```python
from build123d import *

# Parameters (mm, degrees)
SKETCH002_R        = 9.5
SKETCH002_R_2      = 4.05
PAD_DEPTH          = 1
PAD001_DEPTH       = 7
PAD002_DEPTH       = 3
POLARPATTERN_COUNT = 3


with BuildPart() as part:
    # Sketch002 → Pad (new body)
    with BuildSketch(Plane.XY):
        Circle(SKETCH002_R)
        Circle(SKETCH002_R_2, mode=Mode.SUBTRACT)
    extrude(amount=PAD_DEPTH)

    # Sketch003 (on Face4 of Pad) → Pad001 (join)
    with BuildSketch(Plane.XY.offset(1)):
        with BuildLine():
            ThreePointArc((4.0493831654, 0.0706822461), (3.5759377511, 1.9013598293), (2.3229845672, 3.3175657794))
            Line((5.4489761453, 7.7819444208), (2.3229845672, 3.3175657794))
            ThreePointArc((9.498553104, 0.1657978612), (8.3880021321, 4.4599798465), (5.4489761453, 7.7819444208))
            Line((4.0493831654, 0.0706822461), (9.498553104, 0.1657978612))
        make_face()
    pad001 = extrude(amount=PAD001_DEPTH)

    # Sketch004 (on Face8 of Pad001) → Pad002 (join)
    with BuildSketch(Plane.XY.offset(8)):
        Polygon((9.2761791703, 2.05), (10.2761791703, 2.15), (11.2761791703, 1.75), (11.2761791703, -1.75), (10.2761791703, -2.15), (9.2761791703, -2.05), (7.6151685504, 0.1329232615), align=None)
    pad002 = extrude(amount=-PAD002_DEPTH)

    # PolarPattern: Pad001, Pad002 ×3 about axis
    polarpattern_axis = Axis((0, 0, 1), (0, 0, 1))
    for i in range(1, POLARPATTERN_COUNT):
        add(pad001.rotate(polarpattern_axis, i * 360 / POLARPATTERN_COUNT))
        add(pad002.rotate(polarpattern_axis, i * 360 / POLARPATTERN_COUNT))

    # Sketch005 → Groove (revolve, cut)
    with BuildSketch(Plane.XZ):
        Polygon((3.0493831654, 11.2253084173), (3.0493831654, 6), (7.2746915827, 10.2253084173), (12.2761791703, 5.2238208297), (12.2761791703, 11.2253084173), align=None)
    revolve(axis=Axis((0, 0, 0), (0, 0, 1)), mode=Mode.SUBTRACT)


solid = part.part
```
The model under review builds one solid part; all positions refer to its coordinate system, in mm. A direction names the side the tool comes from. Round coordinates to 2 decimals unless told otherwise and drop trailing zeros. Write each loop counter-clockwise with the first axis right and the second up, starting at its lowest first coordinate (ties: lowest second). Pieces come first, ordered by that corner, then holes. Notation, with made-up numbers: M -28,54.25 L -4,54.25 A15 cw -4,70.25 Z; hole C -35.75,49 d1. An arc over 180 degrees is marked long. Use CSV: the item, a comma, the result in double quotes. Start each with the question number.
(1) Tool access review of faces 4 (the face through (2.879, -6.175, 4.451)), 5 (the face through (-6.787, 0.594, 4.451)), 6 (the face through (-5, 9, 5)), 7 (the face through (9.77, 2.1, 6.19)): name each direction out of +Z, -Z, +X, -X, +Y, -Y from which nothing blocks a thin tool from reaching the whole face with its end or side.
(2) We need section B-B, the plane z = 5.25. State how many separate pieces and enclosed holes the cut face has, then the cut area to 3 significant figures.
(3) For line 1 along Y through (x, z) = (0, 0.45); line 2 along Z through (x, y) = (-4.5, -7), list the stretches that pass through material, from the lowest coordinate up.
(4) We need section C-C, the plane y = -5.75. State the section outline as (x, z) points.
(5) We need section D-D, the plane x = 7.25. State the section outline as (y, z) points.
(6) The part is to be moulded in two halves that separate along X. For faces 1 (the face through (-3.754, 2.381, 7.396)), 2 (the face through (-5.659, 9.753, 5.62)), 3 (the face through (11.276, 0, 6)), say which applies: +X half, -X half, draft (parallel to the pull), parting line (faces both ways), or undercut.
(7) Clearance check with flat-ended pins moving along their axes: P1, Ø4, axis at x = 8.5, z = 2, coming from the -Y side; P2, Ø4, axis at y = 5.5, z = 6, coming from the +X side; P3, Ø6.5, axis at x = 0, y = 0, coming from the -Z side; P4, Ø3, axis at y = 8.5, z = 7, coming from the +X side. State where each tip first meets the part, or that it passes through.
(8) We need section A-A, the plane x = 0. State the section outline as (y, z) points, then the cut area to 3 significant figures.
Findings:
1,face 4,"+Z, +X"
1,face 5,"+Z, -X"
1,face 6,"+Y"
1,face 7,"+Z, -Z, +Y"
2,separate pieces,"3"
2,enclosed holes,"0"
2,area,"133 mm^2"
3,line 1,"-9.5 to -4.05, 4.05 to 9.5"
3,line 2,"0 to 1, 5 to 8"
4,outline,"M -7.56,0 L 7.56,0 L 7.56,1 L 2.68,1 L 2.68,8 L -3.19,8 L -3.19,1 L -7.56,1 Z"
5,outline,"M -6.14,0 L 6.14,0 L 6.14,8 L 0.13,8 L 0.13,1 L -6.14,1 Z"
6,face 1,"undercut"
6,face 2,"-X half"
6,face 3,"+X half"
7,P1,"y = -6.67"
7,P2,"x = 8.83"
7,P3,"through"
7,P4,"x = 6.42"
8,outline,"M -9.5,0 L -4.05,0 L -4.05,7 L -5.05,8 L -9.5,8 Z; M 4.05,0 L 9.5,0 L 9.5,1 L 4.05,1 Z"
8,area,"48.6 mm^2"
